Geometry check sheet. Reference: drawing and pictorial views, mm from the part's lowest x, y, z. Coordinates: 2 decimals unless noted, no trailing zeros. Loops run counter-clockwise (first coordinate to the right, second up) from the corner with the lowest first, then second, coordinate; pieces in that order, holes last. Notation, with made-up numbers: (25.5, 34.25) -> (57.5, 34.25) arc R9 cw to (57.5, 41.25) -> close; hole circle Ø9 at (-19, 74.25). An arc over 180 degrees is marked (long way). Use one line per item in the form item = value.
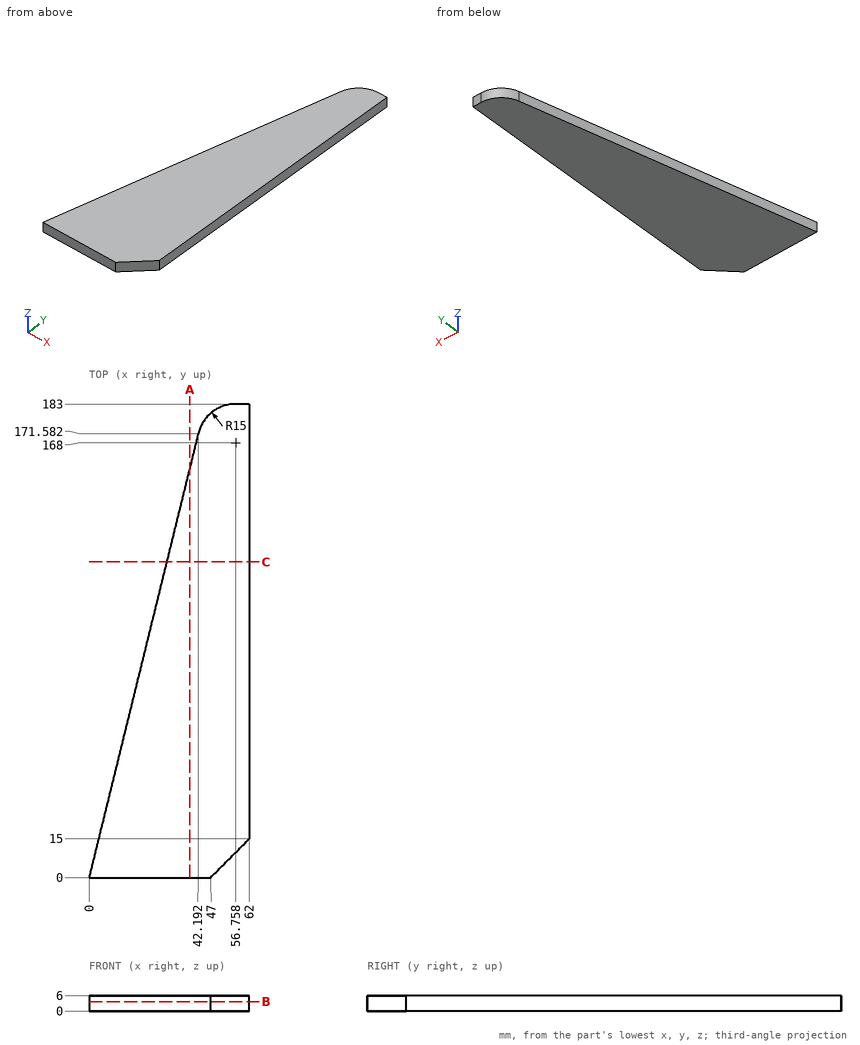
(1) Section check C-C, the plane y = 122. Record the boundary of the cut face in (x, z), plus the area to 3 significant figures.
Established:
outline = (30, 0) -> (62, 0) -> (62, 6) -> (30, 6) -> close
area = 192 mm²
(2) Section check B-B, the plane z = 3.7. Record the boundary of the cut face in (x, y), plus the area to 3 significant figures.
Established:
outline = (0, 0) -> (47, 0) -> (62, 15) -> (62, 183) -> (56.76, 183) arc R15 ccw to (42.19, 171.58) -> close
area = 7,090 mm²
(3) Go/stop test with a flat-tipped pin: P1, Ø4, axis at x = 36, y = 116.5, coming from the -Z side. Record where the tip stops, or that it passes through.
Established:
P1 = 0
(4) Scan lines: line 1 along X through (y, z) = (142.5, 1.3); line 2 along X through (y, z) = (173.5, 3.25); line 3 along Y through (x, z) = (44.5, 2.25) (1 decimal). Record each from-to range of solid material in increasing order.
Established:
line_1 = 35.04 to 62
line_2 = 42.8 to 62
line_3 = 0 to 176.6
(5) Section check A-A, the plane x = 39. Record the boundary of the cut face in (y, z).
Established:
outline = (0, 0) -> (158.6, 0) -> (158.6, 6) -> (0, 6) -> close
